```python
from build123d import *

# Parameters (mm, degrees)
SKETCH004_W     = 48
SKETCH004_H     = 75
SKETCH004_W_2   = 43
SKETCH004_H_2   = 70
PAD002_DEPTH    = 15
SKETCH005_W     = 45.5
SKETCH005_H     = 72.5
POCKET_DEPTH    = 2
FILLET_R        = 3
FILLET001_R     = 3
FILLET002_R     = 3
FILLET003_R     = 3
FILLET004_R     = 3
FILLET005_R     = 3
SKETCH006_W     = 5
SKETCH006_H     = 5
POCKET001_DEPTH = 1
SKETCH007_W     = 5
SKETCH007_H     = 3
POCKET002_DEPTH = 2
SKETCH008_W     = 5
SKETCH008_H     = 5
POCKET003_DEPTH = 1
SKETCH009_W     = 5
SKETCH009_H     = 3
POCKET004_DEPTH = 2
SKETCH011_W     = 23
SKETCH011_H     = 12
POCKET006_DEPTH = 2
SKETCH013_W     = 8
SKETCH013_H     = 5
POCKET008_DEPTH = 5


with BuildPart() as part:
    # Sketch004 → Pad002 (new body)
    with BuildSketch(Plane.XY.offset(1.5)):
        with Locations((-5, 0)):
            Rectangle(SKETCH004_W, SKETCH004_H)
        with Locations((-5, 0)):
            Rectangle(SKETCH004_W_2, SKETCH004_H_2, mode=Mode.SUBTRACT)
    extrude(amount=PAD002_DEPTH)

    # Sketch005 → Pocket (cut)
    with BuildSketch(Plane.XY.offset(16.5)):
        with Locations((-4.9611, 0)):
            Rectangle(SKETCH005_W, SKETCH005_H)
    extrude(amount=-POCKET_DEPTH, mode=Mode.SUBTRACT)

    # Fillet
    fillet_edges = [part.edges().sort_by_distance(p)[0] for p in [
        (-27.7111, 36.25, 15.5),
    ]]
    fillet(fillet_edges, radius=FILLET_R)

    # Fillet001
    fillet001_edges = [part.edges().sort_by_distance(p)[0] for p in [
        (-27.7111, -36.25, 15.5),
    ]]
    fillet(fillet001_edges, radius=FILLET001_R)

    # Fillet002
    fillet002_edges = [part.edges().sort_by_distance(p)[0] for p in [
        (17.7889, -36.25, 15.5),
    ]]
    fillet(fillet002_edges, radius=FILLET002_R)

    # Fillet003
    fillet003_edges = [part.edges().sort_by_distance(p)[0] for p in [
        (17.7889, 36.25, 15.5),
    ]]
    fillet(fillet003_edges, radius=FILLET003_R)

    # Fillet004
    fillet004_edges = [part.edges().sort_by_distance(p)[0] for p in [
        (-29, 37.5, 9),
        (19, 37.5, 9),
    ]]
    fillet(fillet004_edges, radius=FILLET004_R)

    # Fillet005
    fillet005_edges = [part.edges().sort_by_distance(p)[0] for p in [
        (-29, -37.5, 9),
        (19, -37.5, 9),
    ]]
    fillet(fillet005_edges, radius=FILLET005_R)

    # Sketch006 → Pocket001 (cut)
    with BuildSketch(Plane(origin=(-26.5, 0, 1.5), x_dir=(0, 1, 0), z_dir=(1, 0, 0))):
        with Locations((0, 10.5)):
            Rectangle(SKETCH006_W, SKETCH006_H)
    extrude(amount=-POCKET001_DEPTH, mode=Mode.SUBTRACT)

    # Sketch007 → Pocket002 (cut)
    with BuildSketch(Plane(origin=(-26.5, 0, 1.5), x_dir=(0, 1, 0), z_dir=(1, 0, 0))):
        with Locations((0, 6.5)):
            Rectangle(SKETCH007_W, SKETCH007_H)
    extrude(amount=-POCKET002_DEPTH, mode=Mode.SUBTRACT)

    # Sketch008 → Pocket003 (cut)
    with BuildSketch(Plane(origin=(16.5, 0, 1.5), x_dir=(0, -1, 0), z_dir=(-1, 0, 0))):
        with Locations((0, 10.5)):
            Rectangle(SKETCH008_W, SKETCH008_H)
    extrude(amount=-POCKET003_DEPTH, mode=Mode.SUBTRACT)

    # Sketch009 → Pocket004 (cut)
    with BuildSketch(Plane(origin=(16.5, 0, 1.5), x_dir=(0, -1, 0), z_dir=(-1, 0, 0))):
        with Locations((0, 6.5)):
            Rectangle(SKETCH009_W, SKETCH009_H)
    extrude(amount=-POCKET004_DEPTH, mode=Mode.SUBTRACT)

    # Sketch011 → Pocket006 (cut)
    with BuildSketch(Plane(origin=(0, -35, 1.5), x_dir=(-1, 0, 0), z_dir=(0, 1, 0))):
        with Locations((0, 6)):
            Rectangle(SKETCH011_W, SKETCH011_H)
    extrude(amount=-POCKET006_DEPTH, mode=Mode.SUBTRACT)

    # Sketch013 → Pocket008 (cut)
    with BuildSketch(Plane(origin=(0, -37.5, 1.5), x_dir=(1, 0, 0), z_dir=(0, -1, 0))):
        with Locations((0, 9.5)):
            Rectangle(SKETCH013_W, SKETCH013_H)
    extrude(amount=-POCKET008_DEPTH, mode=Mode.SUBTRACT)


solid = part.part
```
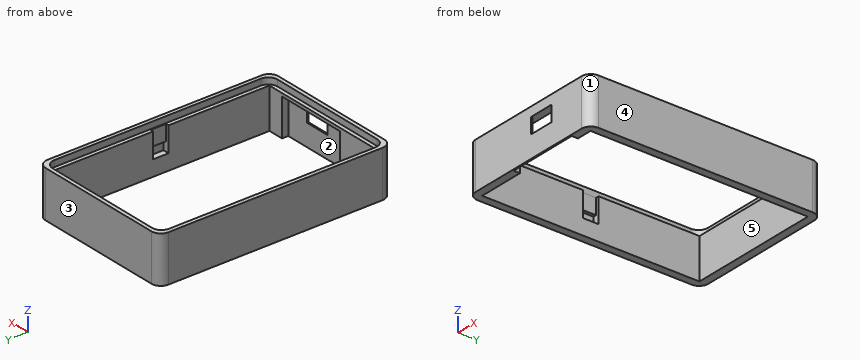
Input: part model. Units: mm. Frame: model coordinates. Face numbers are marked on the shaded views. A direction names the side the tool comes from. Coordinates: 2 decimals unless noted, no trailing zeros. Write each loop counter-clockwise with the first axis right and the second up, starting at its lowest first coordinate (ties: lowest second). Pieces come first, ordered by that corner, then holes. Notation, with made-up numbers: (-11.75, -38.5) - (7.25, -38.5) arc R33 cw to (7.25, -6.5) - close; hole circle Ø5 at (84, 47.25). An arc over 180 degrees is marked (long way). Put each result on its own line as item: value. Start each with the question number.
1) Reachability of the marked faces 4 and 5 from +Z, -Z, +X, -X, +Y, -Y: full face, straight path, thin tool, end or side. Return the list, or none.
2) Mould query, pull axis X, two halves, no side actions, for the marked faces 1, 2 and 3. Classes: pulls with the +X half, pulls with the -X half, needs draft (parallel to the pull), parting line crosses it, or undercut.
3) Ray query, L1, parallel to Y at x = -17, z = 11.5; L2, parallel to Y at x = 10.5, z = 13.25; L3, parallel to X at y = 15, z = 13.5. Return the intervals inside material, ascending.
4) Cut plane B-B (z = 5.5). Return the cut outline in (x, y).
5) Cut plane D-D (x = -2). Return the cut outline in (y, z), plus the area to 3 significant figures.
6) Contact query for flat-ended pins moving along their axis: pin 1 (2 mm diameter, centred on x = -28, z = 10.5, fed in from +Y); pin 2 (0.6 mm diameter, centred on y = -36.5, z = 5.5, fed in from -X); pin 3 (2 mm diameter, centred on x = 17, y = 0, fed in from +Z); pin 4 (1.6 mm diameter, centred on x = 17.5, z = 10.5, fed in from -Y). Output: stop coordinate, or through.
7) Cut plane A-A (x = -15.5). Return the cut outline in (y, z), plus the area to 3 significant figures.
8) Cut plane C-C (y = -18). Return the cut outline in (x, z), plus the area to 3 significant figures.
Resolved:
1. face 4: +Z, -Z, +X, +Y, -Y
1. face 5: +Z, -Z
2. face 1: pulls with the +X half
2. face 2: undercut
2. face 3: needs draft
3. L1: y = -37.5 to -35, 35 to 37.5
3. L2: y = -37.5 to -37, 35 to 37.5
3. L3: x = -29 to -26.5, 16.5 to 19
4. outline: (-29, -34.5) arc R3 ccw to (-26, -37.5) - (16, -37.5) arc R3 ccw to (19, -34.5) - (19, 34.5) arc R3 ccw to (16, 37.5) - (-26, 37.5) arc R3 ccw to (-29, 34.5) - close; hole (-26.5, -35) - (-11.5, -35) - (-11.5, -37) - (11.5, -37) - (11.5, -35) - (16.5, -35) - (16.5, 35) - (-26.5, 35) - close
5. outline: (-37.5, 1.5) - (-37, 1.5) - (-37, 8.5) - (-37.5, 8.5) - close; (-37.5, 13.5) - (-35, 13.5) - (-35, 14.5) - (-36.25, 14.5) - (-36.25, 16.5) - (-37.5, 16.5) - close; (35, 1.5) - (37.5, 1.5) - (37.5, 16.5) - (36.25, 16.5) - (36.25, 14.5) - (35, 14.5) - close
5. area: 43.5 mm2
6. pin 1: stops at y = 37.33
6. pin 2: stops at x = -28.47
6. pin 3: stops at z = 16.5
6. pin 4: stops at y = -37.42
7. outline: (-37.5, 1.5) - (-35, 1.5) - (-35, 14.5) - (-36.25, 14.5) - (-36.25, 16.5) - (-37.5, 16.5) - close; (35, 1.5) - (37.5, 1.5) - (37.5, 16.5) - (36.25, 16.5) - (36.25, 14.5) - (35, 14.5) - close
7. area: 70.0 mm2
8. outline: (-29, 1.5) - (-26.5, 1.5) - (-26.5, 14.5) - (-27.71, 14.5) - (-27.71, 16.5) - (-29, 16.5) - close; (16.5, 1.5) - (19, 1.5) - (19, 16.5) - (17.79, 16.5) - (17.79, 14.5) - (16.5, 14.5) - close
8. area: 70.0 mm2
